Autodesk Inventor part; units mm, degrees
ref_plane "YZ Plane" through (0, 0, 0) normal (1, 0, 0) x (0, 1, 0)
ref_plane "XZ Plane" through (0, 0, 0) normal (0, 1, 0) x (-1, 0, 0)
ref_plane "XY Plane" through (0, 0, 0) normal (0, 0, 1) x (1, 0, 0)
sketch "Sketch1" plane through (0, 0, 0) normal (0, 1, 0) x (-1, 0, 0)
  line L0 (85, 0) -> (85, -112)
  line L1 (85, -112) -> (0, -112)
  line L2 (0, -112) -> (0, 0)
  arc A0 (7.3966, 0) -> (77.6034, 0) centre (42.5, 32) ccw
  line L3 (0, 0) -> (7.3966, 0)
  line L4 (77.6034, 0) -> (85, 0)
  dimension "d0" = 112
  dimension "d1" = 85
extrude "Extrusion1" add sketch "Sketch1" along normal blind 3
properties part number "Electronics Plate"
Geometry: final body of the model. Coordinates: model frame, mm. Round coordinates to 2 decimals unless told otherwise and drop trailing zeros. Loops run counter-clockwise (first coordinate to the right, second up) from the corner with the lowest first, then second, coordinate; pieces in that order, holes last. Notation, with made-up numbers: M -35,38 L -4,38 A23 cw -4,46 Z; hole C 25.5,-18 d5. An arc over 180 degrees is marked long. Put each result on its own line as item: value. Start each with the question number.
(1) Material intervals for line 1 along Z through (x, y) = (-38.5, 0.25); line 2 along Z through (x, y) = (-44.5, 2.05), sorted ascending. Write a range as [from, to].
(2) Section query D-D (x = -52). Return loops of the section in (y, z), then the cut area to 3 significant figures.
(3) Section query B-B (y = 1.65). Return loops of the section in (x, z).
(4) Section query C-C (x = -65). Return loops of the section in (y, z), then the cut area to 3 significant figures.
(5) Draft query along X for faces 1 (the face through (0, 1, -57)), 2 (the face through (-43.053, 1.479, -15.497)), 3 (the face through (-42, 0, -55)). Return one class per face: +X half, -X half, draft (parallel to the pull), parting line (faces both ways), or undercut.
(6) Section query A-A (z = -9). Return loops of the section in (x, y), then the cut area to 3 significant figures.
Findings below:
1. line 1: z = [-112, -15.33]
1. line 2: z = [-112, -15.46]
2. outline: M 0,-112 L 3,-112 L 3,-14.54 L 0,-14.54 Z
2. area: 292 mm2
3. outline: M -85,-112 L 0,-112 L 0,0 L -7.4,0 A47.5 cw -77.6,0 L -85,0 Z
4. outline: M 0,-112 L 3,-112 L 3,-9.83 L 0,-9.83 Z
4. area: 307 mm2
5. face 1: +X half
5. face 2: undercut
5. face 3: draft
6. outline: M -85,0 L -66.48,0 L -66.48,3 L -85,3 Z; M -18.52,0 L 0,0 L 0,3 L -18.52,3 Z
6. area: 111 mm2
